Autodesk Inventor part; units mm, degrees
ref_plane "YZ Plane" through (0, 0, 0) normal (1, 0, 0) x (0, 1, 0)
ref_plane "XZ Plane" through (0, 0, 0) normal (0, 1, 0) x (-1, 0, 0)
ref_plane "XY Plane" through (0, 0, 0) normal (0, 0, 1) x (1, 0, 0)
sketch "Sketch1" plane through (0, 0, 0) normal (0, 1, 0) x (-1, 0, 0)
  line L0 (7.7899, 9.4408) -> (-35.6101, 9.4408)
  line L1 (-35.6101, 9.4408) -> (-35.6101, -11.1592)
  line L2 (-35.6101, -11.1592) -> (7.7899, -11.1592)
  line L3 (7.7899, -11.1592) -> (7.7899, 9.4408)
  point P0 (0, 0)
  dimension "d0" = 43.4
  dimension "d1" = 20.6
extrude "Extrusion1" add sketch "Sketch1" along normal blind 1.2
sketch "Sketch2" plane through (0, 1.2, 0) normal (0, 1, 0) x (1, 0, 0)
  circle A0 centre (31.6101, 1.1592) radius 4
  line L0 (35.6101, 11.1592) -> (-7.7899, 11.1592)
  circle A1 centre (-3.7899, 1.1592) radius 4
  line L1 (-7.7899, 11.1592) -> (-7.7899, -9.4408)
  line L2 (35.6101, -9.4408) -> (35.6101, 11.1592)
  point P0 (0, 0)
  dimension "d4" = 8
  dimension "d5" = 10
  dimension "d6" = 8
  dimension "d7" = 4
  dimension "d8" = 4
extrude "Extrusion2" add sketch "Sketch2" along normal blind 12
fillet "Fillet1" radius 0.5 2 edges at (27.6101, 13.2, -1.1592) (-7.7899, 13.2, -1.1592)
sketch "Sketch3" plane through (0, 1.2, 0) normal (0, 1, 0) x (1, 0, 0)
  line L0 (9.4101, -5.0408) -> (-0.1899, -5.0408)
  line L1 (-0.1899, -5.0408) -> (-0.1899, -9.4408)
  line L2 (-0.1899, -9.4408) -> (9.4101, -9.4408)
  line L3 (9.4101, -9.4408) -> (9.4101, -5.0408)
  line L4 (-7.7899, -9.4408) -> (35.6101, -9.4408)
  line L5 (-7.7899, 1.1592) -> (-7.7899, -9.4408)
  point P0 (0, 0)
  dimension "d12" = 9.6
  dimension "d13" = 4.4
  dimension "d14" = 0
  dimension "d15" = 7.6
extrude "Extrusion3" add sketch "Sketch3" along normal blind 10.1
sketch "Sketch4" plane through (0, 1.2, 0) normal (0, 1, 0) x (1, 0, 0)
  circle A0 centre (28.5101, -6.7408) radius 1.5
  line L0 (35.6101, -9.4408) -> (35.6101, 1.1592)
  line L1 (-7.7899, -9.4408) -> (35.6101, -9.4408)
  circle A1 centre (-1.2899, 8.4592) radius 1.5
  line L2 (35.6101, 11.1592) -> (-7.7899, 11.1592)
  line L3 (-7.7899, 11.1592) -> (-7.7899, -9.4408)
  point P0 (0, 0)
  dimension "d18" = 3
  dimension "d19" = 7.1
  dimension "d20" = 2.7
  dimension "d21" = 3
  dimension "d22" = 2.7
  dimension "d23" = 6.5
extrude "Extrusion4" cut sketch "Sketch4" against normal blind 10.1
sketch "Sketch5" plane through (0, 1.2, 0) normal (0, 1, 0) x (1, 0, 0)
  line L0 (14.4101, -1.8408) -> (2.2101, -1.8408)
  line L1 (2.2101, -1.8408) -> (2.2101, 10.3592)
  line L2 (2.2101, 10.3592) -> (14.4101, 10.3592)
  line L3 (14.4101, 10.3592) -> (14.4101, -1.8408)
  line L4 (35.6101, 11.1592) -> (-7.7899, 11.1592)
  line L5 (-7.7899, 11.1592) -> (-7.7899, 1.1592)
  point P0 (0, 0)
  dimension "d26" = 12.2
  dimension "d27" = 12.2
  dimension "d28" = 0.8
  dimension "d29" = 10
extrude "Extrusion5" add sketch "Sketch5" along normal blind 7.2
sketch "Sketch6" plane through (0, 1.2, 0) normal (0, 1, 0) x (1, 0, 0)
  line L0 (25.6101, 2.9592) -> (15.6101, 2.9592)
  line L1 (15.6101, 2.9592) -> (15.6101, -5.4408)
  line L2 (15.6101, -5.4408) -> (25.6101, -5.4408)
  line L3 (25.6101, -5.4408) -> (25.6101, 2.9592)
  line L4 (9.4101, -9.4408) -> (35.6101, -9.4408)
  line L5 (35.6101, -9.4408) -> (35.6101, 1.1592)
  point P0 (0, 0)
  dimension "d32" = 10
  dimension "d33" = 8.4
  dimension "d34" = 4
  dimension "d35" = 10
extrude "Extrusion6" add sketch "Sketch6" along normal blind 4.4
sketch "Sketch7" plane through (0, 1.2, 0) normal (0, 1, 0) x (1, 0, 0)
  circle A0 centre (28.5101, -6.7408) radius 1.5
  circle A1 centre (28.5101, -6.7408) radius 1.5
  circle A2 centre (-1.2899, 8.4592) radius 1.5
  circle A3 centre (-1.2899, 8.4592) radius 1.5
  point P0 (0, 0)
properties part number "DC menic"
Work out the finished part from the listing and answer in its coordinate system (mm). A direction names the side the tool comes from. Round coordinates to 2 decimals unless told otherwise and drop trailing zeros. Loops run counter-clockwise (first coordinate to the right, second up) from the corner with the lowest first, then second, coordinate; pieces in that order, holes last. Notation, with made-up numbers: M 34,64.25 L 84,64.25 A6 ccw 84,72.25 Z; hole C 30,5 d4. An arc over 180 degrees is marked long. One line per question, with ' | ' between items.
Q1. Find section D-D, the plane y = 4. Give the vertices of the cut face in (x, z).
Conclusion:
outline: C -3.79,-1.16 d8; M -0.19,5.04 L 9.41,5.04 L 9.41,9.44 L -0.19,9.44 Z; M 2.21,-10.36 L 14.41,-10.36 L 14.41,1.84 L 2.21,1.84 Z; M 15.61,-2.96 L 25.61,-2.96 L 25.61,5.44 L 15.61,5.44 Z; C 31.61,-1.16 d8
Q2. The mould has two halves that part along X. Classify faces 6 (the flat face through (5, 11.3, 7)), 7 (the flat face through (35.61, 1, -1)), 8 (the flat face through (2.21, 5, -4)): +X half, -X half, draft (parallel to the pull), parting line (faces both ways), or undercut.
Conclusion:
face 6: draft | face 7: +X half | face 8: undercut
Q3. Find section C-C, the plane x = 22. Give the vertices of the cut face in (y, z), then the cut area to 3 significant figures.
Conclusion:
outline: M 0,-11.16 L 1.2,-11.16 L 1.2,-2.96 L 5.6,-2.96 L 5.6,5.44 L 1.2,5.44 L 1.2,9.44 L 0,9.44 Z | area: 61.7 mm2
Q4. A tool of negligible diameter and unlimited length cuts with its end or side. For faces 1 (the flat face through (21, 3, 5.441)), 2 (the flat face through (8, 5, -10.359)), 3 (the flat face through (5, 6, 5.041)), 4 (the flat face through (25.61, 3, 1)), 5 (the cylindrical face through (0.025, 6.87, 0.042)), from which of +Z, -Z, +X, -X, +Y, -Y can it reach the whole face along a straight path? Write none if from no direction.
Conclusion:
face 1: +Z, +X, +Y | face 2: -Z, +X, -X, +Y | face 3: -X, +Y | face 4: +Z, -Z, +Y | face 5: +Y
Q5. Find section A-A, the plane y = 6. Give the vertices of the cut face in (x, z).
Conclusion:
outline: C -3.79,-1.16 d8; M -0.19,5.04 L 9.41,5.04 L 9.41,9.44 L -0.19,9.44 Z; M 2.21,-10.36 L 14.41,-10.36 L 14.41,1.84 L 2.21,1.84 Z; C 31.61,-1.16 d8
Q6. Each of these flat-tipped pins is pushed along its axis until it touches: pin 1 Ø3.5 at (x, y) = (11, 6) entering from -Z; pin 2 Ø1.5 at (x, z) = (21, 6) entering from +Y; pin 3 Ø5 at (y, z) = (4, 2.5) entering from -X. Where does it stop, or does it pass through?
Conclusion:
pin 1: stops at z = -10.36 | pin 2: stops at y = 5.6 | pin 3: stops at x = -7.62
Q7. Find section B-B, the plane z = -6. Give the vertices of the cut face in (x, y).
Conclusion:
outline: M -7.79,0 L 35.61,0 L 35.61,1.2 L 14.41,1.2 L 14.41,8.4 L 2.21,8.4 L 2.21,1.2 L -7.79,1.2 Z
Q8. Consider line 1 along X through (y, z) = (4.75, 0); line 2 along X through (y, z) = (2, -2); line 3 along Z through (x, y) = (1.5, 4). Determine where each line is inside the solid, lowest interval first. Write a range as from..to.
Conclusion:
line 1: x = -7.62..0.04, 2.21..14.41, 15.61..25.61, 27.78..35.44 | line 2: x = -7.7..0.12, 2.21..14.41, 15.61..25.61, 27.7..35.52 | line 3: z = 5.04..9.44
